Verification items for the finished model (mm, model axes). A direction names the side the tool comes from. Round coordinates to 2 decimals unless told otherwise and drop trailing zeros. Write each loop counter-clockwise with the first axis right and the second up, starting at its lowest first coordinate (ties: lowest second). Pieces come first, ordered by that corner, then holes. Notation, with made-up numbers: M 72.5,45 L 81.5,45 A19 cw 81.5,78 Z; hole C -14,42.5 d11. An arc over 180 degrees is marked long. Answer in a Markdown table with one row per item. Add a question column.
1. Sectioned sample at A-A on x = -54. Record the cut outline in (y, z).
2. Material ranges on probe 1 along Y at (x, z) = (-239.5, -72); probe 2 along Z at (x, y) = (-150.5, 460); probe 3 along X at (y, z) = (964.5, -105), recorded low to high.
3. Sectioned sample at B-B on z = -12. Record the cut outline in (x, y), plus the area to 3 significant figures.
4. Sectioned sample at C-C on x = -198.5. Record the cut outline in (y, z).
5. Set-up check for faces 4 (the flat face through (-185, 1174, 111.848)), 5 (the cylindrical face through (-99.14, 589.08, -103.45)), 6 (the flat face through (-175, 589, -64.513)), 7 (the flat face through (-185, 19, -296.455)), 8 (the cylindrical face through (-251.523, 589.077, -101.776)): record each of +Z, -Z, +X, -X, +Y, -Y from which the full face is reachable in a straight line by a thin tool's end or side.
6. Sectioned sample at D-D on z = -100. Record the cut outline in (x, y).
7. Draft check along Y on faces 1 (the flat face through (-176, 589, -140.713)), 2 (the flat face through (-185, 1193.8, -101)), 3 (the flat face through (-391.773, 19, -84)). Enter one of: pulls with the +Y half, pulls with the -Y half, needs draft (parallel to the pull), parting line crosses it, or undercut.
8. Go/stop test with flat-tipped pins: pin 1 Ø8 at (x, y) = (-102, 765) entering from -Z; pin 2 Ø23 at (x, y) = (-181, 737) entering from +Z; pin 3 Ø1.5 at (x, y) = (-130, 312) entering from -Z. Record where each tip stops, or that it passes through.
```python
from build123d import *

# Parameters (mm, degrees)
SKETCH1_W           = 419.1
SKETCH1_H           = 419.1
BOSS_EXTRUDE1_DEPTH = 38.1
BOSS_EXTRUDE2_DEPTH = 1117.6
SKETCH6_W           = 419.1
SKETCH6_H           = 419.1
BOSS_EXTRUDE4_DEPTH = 38.1


with BuildPart() as part:
    # Sketch1 → Boss-Extrude1 (new body)
    with BuildSketch(Plane(origin=(0, 0, 0), x_dir=(1, 0, 0), z_dir=(0, 1, 0))):
        with Locations((-182.222860504, 86.904880256)):
            Rectangle(SKETCH1_W, SKETCH1_H)
    extrude(amount=BOSS_EXTRUDE1_DEPTH)

    # Sketch4 → Boss-Extrude2 (add)
    with BuildSketch(Plane(origin=(0, 38.1, 0), x_dir=(1, 0, 0), z_dir=(0, 1, 0))):
        with BuildLine():
            Line((-213.432103513, 140.713298357), (-137.232103513, 140.713298357))
            ThreePointArc((-137.232103513, 140.713298357), (-99.132103513, 102.613298357), (-137.232103513, 64.513298357))
            Line((-137.232103513, 64.513298357), (-213.432103513, 64.513298357))
            ThreePointArc((-213.432103513, 64.513298357), (-251.532103513, 102.613298357), (-213.432103513, 140.713298357))
        make_face()
    extrude(amount=BOSS_EXTRUDE2_DEPTH)

    # Sketch6 → Boss-Extrude4 (add)
    with BuildSketch(Plane(origin=(0, 1155.7, 0), x_dir=(1, 0, 0), z_dir=(0, 1, 0))):
        with Locations((-182.168261088, 97.701559628)):
            Rectangle(SKETCH6_W, SKETCH6_H)
    extrude(amount=BOSS_EXTRUDE4_DEPTH)


solid = part.part
```
Geometry check:
| question | item | result |
|---|---|---|
| 1 | outline | M 0,-296.45 L 38.1,-296.45 L 38.1,122.65 L 0,122.65 Z; M 1155.7,-307.25 L 1193.8,-307.25 L 1193.8,111.85 L 1155.7,111.85 Z |
| 2 | probe 1 | y = 0 to 38.1, 1155.7 to 1193.8 |
| 2 | probe 2 | z = -140.71 to -64.51 |
| 2 | probe 3 | x = -251.46 to -99.21 |
| 3 | outline | M -391.77,0 L 27.33,0 L 27.33,38.1 L -391.77,38.1 Z; M -391.72,1155.7 L 27.38,1155.7 L 27.38,1193.8 L -391.72,1193.8 Z |
| 3 | area | 31,900 mm2 |
| 4 | outline | M 0,-296.45 L 38.1,-296.45 L 38.1,-140.71 L 1155.7,-140.71 L 1155.7,-307.25 L 1193.8,-307.25 L 1193.8,111.85 L 1155.7,111.85 L 1155.7,-64.51 L 38.1,-64.51 L 38.1,122.65 L 0,122.65 Z |
| 5 | face 4 | +Z, +X, -X, +Y |
| 5 | face 5 | +X |
| 5 | face 6 | +Z, +X, -X |
| 5 | face 7 | -Z, +X, -X, -Y |
| 5 | face 8 | -X |
| 6 | outline | M -391.77,0 L 27.33,0 L 27.33,38.1 L -99.22,38.1 L -99.22,1155.7 L 27.38,1155.7 L 27.38,1193.8 L -391.72,1193.8 L -391.72,1155.7 L -251.44,1155.7 L -251.44,38.1 L -391.77,38.1 Z |
| 7 | face 1 | undercut |
| 7 | face 2 | pulls with the +Y half |
| 7 | face 3 | needs draft |
| 8 | pin 1 | stops at z = -124.43 |
| 8 | pin 2 | stops at z = -64.51 |
| 8 | pin 3 | stops at z = -140.16 |
